Here's how the part is built. I have some questions about the finished solid (model axes, mm). Face numbers are marked on the shaded views. A direction names the side the tool comes from. Round coordinates to 2 decimals unless told otherwise and drop trailing zeros. Order: outer loops, then holes, each group sorted by start corner. A loop starts at its lowest first (then second) coordinate and runs counter-clockwise, first axis right, second up. Notation, with made-up numbers: (54.5, 69) -> (63.5, 69) arc R15 ccw to (63.5, 88) -> close; hole circle Ø5 at (11.25, 53.25). An arc over 180 degrees is marked (long way). One line per item, written item: value.
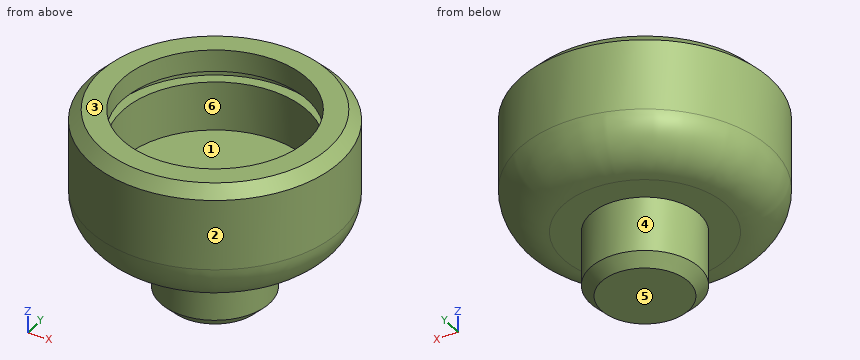
Autodesk Inventor part; units mm, degrees
ref_plane "YZ Plane" through (0, 0, 0) normal (1, 0, 0) x (0, 1, 0)
ref_plane "XZ Plane" through (0, 0, 0) normal (0, 1, 0) x (-1, 0, 0)
ref_plane "XY Plane" through (0, 0, 0) normal (0, 0, 1) x (1, 0, 0)
sketch "Boceto1" plane through (0, 0, 0) normal (0, 1, 0) x (-1, 0, 0)
  line L0 (0, 0) -> (17, 0) construction
  line L1 (17, -15) -> (0, -15)
  line L2 (0, -15) -> (0, -35)
  line L3 (0, -35) -> (8, -35)
  line L4 (10, -33) -> (10, -23)
  line L5 (10, -23) -> (15, -23)
  line L6 (23, -15) -> (23, -2)
  line L7 (8, -35) -> (10, -33)
  arc A0 (15, -23) -> (23, -15) centre (15, -15) ccw
  line L8 (21, 0) -> (17, 0)
  line L9 (23, -2) -> (21, 0)
  line L10 (17, 0) -> (17, -4) construction
  line L11 (17, -4) -> (19, -4)
  line L12 (19, -4) -> (19, -6)
  line L13 (19, -6) -> (17, -6)
  line L14 (17, 0) -> (17, -4)
  line L15 (17, -6) -> (17, -15)
  point P0 (10, -35)
  point P1 (23, 0)
  point P2 (23, 0)
  dimension "d2" = 17
  dimension "d4" = 2
  dimension "d5" = 45
  dimension "d11" = 8
  dimension "d13" = 23
  dimension "d14" = 10
  dimension "d15" = 10
  dimension "d17" = 15
  dimension "d18" = 2
  dimension "d19" = 45
  dimension "d20" = 35
  dimension "d21" = 4
  dimension "d22" = 2
  dimension "d23" = 2
  dimension "d24" = 9
revolve "Revolución1" add sketch "Boceto1" angle 360 about axis through (0, 0, -15) along (0, 0, -1)
equation "\"Radio_pliegue\" = Grosor"
equation "\"Anchura_desahogo_plegado\" = Grosor"
equation "\"Profundidad_desahogo_plegado\" = 0.5 * Grosor"
equation "\"Tamaño_destalonado\" = 4 * Grosor"
equation "\"Remanente_mínimo\" = 2 * Grosor"
equation "\"Radiodetransición\" = Radio_pliegue"
equation "\"Tamaño_de_radio_de_Jacobi\" = Radio_pliegue"
equation "\"TamañoSeparación\" = Grosor"
properties part number "Practica 5"
Q1. For P1, Ø1.5, axis at x = -8.5, y = 11.5, coming from the -Z side; P2, Ø1, axis at x = 10, z = -17, coming from the +Y side; P3, Ø5, axis at y = 6, z = -20.5, coming from the +X side, each with a flat end and sliding along its axis, tell me the tip position at first contact or that it passes through.
Answers:
P1: z = -23
P2: y = 20.7
P3: x = 21.76
Q2. Which directions (+Z, -Z, +X, -X, +Y, -Y) give clear straight access to the entire face, cutting with the end or side of a thin tool? Please do the marked faces 4, 5 and 6.
Answers:
face 4: -Z
face 5: -Z, +X, -X, +Y, -Y
face 6: +Z
Q3. I want a section at C-C on z = -28. Write out the boundary of the cut face in (x, y).
Answers:
outline: circle Ø20 at (0, 0)
Q4. I want a section at D-D on z = -18. Write out the boundary of the cut face in (x, y), then the cut area to 3 significant figures.
Answers:
outline: circle Ø44.83 at (0, 0)
area: 1,580 mm2
Q5. If we mould it in two halves opening along X, with no side actions, what happens to the marked faces 1, 2 and 3? For each: pulls with the +X half, pulls with the -X half, needs draft (parallel to the pull), parting line crosses it, or undercut.
Answers:
face 1: undercut
face 2: parting line crosses it
face 3: needs draft
Q6. I want a section at A-A on y = 0. Write out the boundary of the cut face in (x, z), then the cut area to 3 significant figures.
Answers:
outline: (-23, -15) arc R8 ccw to (-15, -23) -> (-10, -23) -> (-10, -33) -> (-8, -35) -> (8, -35) -> (10, -33) -> (10, -23) -> (15, -23) arc R8 ccw to (23, -15) -> (23, -2) -> (21, 0) -> (17, 0) -> (17, -4) -> (19, -4) -> (19, -6) -> (17, -6) -> (17, -15) -> (-17, -15) -> (-17, -6) -> (-19, -6) -> (-19, -4) -> (-17, -4) -> (-17, 0) -> (-21, 0) -> (-23, -2) -> close
area: 745 mm2
Q7. I need wall thicknesses on line 1 along Y through (x, z) = (0, -2.1); line 2 along Z through (x, y) = (5, 3); line 3 along Y through (x, z) = (3.5, -2). Which ranges of each line are inside material? Lowest first, please.
Answers:
line 1: -23 to -17, 17 to 23
line 2: -35 to -15
line 3: -22.73 to -16.64, 16.64 to 22.73
